CAD build for the part. Positions are in the model's coordinates, mm. Face numbers are marked on the shaded views. A direction names the side the tool comes from. Coordinates: 2 decimals unless noted, no trailing zeros. Order: outer loops, then holes, each group sorted by start corner. A loop starts at its lowest first (then second) coordinate and runs counter-clockwise, first axis right, second up. Notation, with made-up numbers: M 56,-24 L 71,-24 A32 cw 71,2 Z; hole C 89.25,-21 d5. An arc over 180 degrees is marked long. One line per item, written item: value.
Autodesk Inventor part; units mm, degrees
ref_plane "YZ Plane" through (0, 0, 0) normal (1, 0, 0) x (0, 1, 0)
ref_plane "XZ Plane" through (0, 0, 0) normal (0, 1, 0) x (-1, 0, 0)
ref_plane "XY Plane" through (0, 0, 0) normal (0, 0, 1) x (1, 0, 0)
sketch "Sketch1" plane through (0, 0, 0) normal (0, 0, 1) x (1, 0, 0)
  line L0 (0, 0) -> (82.55, 0)
  line L1 (82.55, 0) -> (82.55, 123.825)
  line L2 (82.55, 123.825) -> (0, 123.825)
  line L3 (0, 123.825) -> (0, 0)
  arc A0 (73.025, 123.825) -> (0, 6.35) centre (216.4664, -46.7758) ccw
  point P0 (60.325, 123.825)
  dimension "d0" = 82.55
  dimension "d1" = 123.825
  dimension "d5" = 9.525
  dimension "d6" = 6.35
extrude "Extrusion1" add sketch "Sketch1" along normal mid plane 46.0375 contours L3 A0 L2 L1 L0
sketch "Sketch3" plane through (0, 0, 23.0187) normal (-1, 0, 0) x (0, 0, 1)
  line L0 (-39.6875, 117.475) -> (-6.35, 117.475)
  line L1 (-6.35, 117.475) -> (-6.35, 3.175)
  line L2 (-6.35, 3.175) -> (-39.6875, 3.175)
  line L3 (-39.6875, 3.175) -> (-39.6875, 117.475)
  line L4 (0, 6.35) -> (0, 123.825)
  line L5 (-46.0375, 123.825) -> (0, 123.825)
  point P0 (-23.0187, 0)
  dimension "d9" = 33.3375
  dimension "d10" = 114.3
  dimension "d11" = 6.35
  dimension "d12" = 6.35
extrude "Extrusion2" cut sketch "Sketch3" along normal mid plane 158.75
sketch "Sketch4" plane through (79.375, 0, 23.0187) normal (-1, 0, 0) x (0, 0, 1)
  line L0 (-39.6875, 117.475) -> (-6.35, 117.475)
  line L1 (-39.6875, 117.475) -> (-6.35, 117.475)
  line L2 (-23.0188, 117.475) -> (-23.0188, 92.075)
  line L3 (-29.3688, 98.425) -> (-16.6688, 98.425)
  line L4 (-16.6688, 98.425) -> (-16.6688, 85.725)
  line L5 (-16.6688, 85.725) -> (-29.3688, 85.725)
  line L6 (-29.3688, 85.725) -> (-29.3688, 98.425)
  line L7 (-29.3688, 98.425) -> (-16.6688, 85.725) construction
  line L8 (-16.6688, 98.425) -> (-29.3688, 85.725) construction
  point P0 (-23.0187, 0)
  dimension "d26" = 25.4
  dimension "d27" = 12.7
  dimension "d28" = 12.7
extrude "Extrusion3" cut sketch "Sketch4" against normal through all
sketch "Sketch5" plane through (0, 3.175, 16.6688) normal (0, 1, 0) x (1, 0, 0)
  line L0 (60.325, 26.9875) -> (22.225, 26.9875)
  line L1 (22.225, 26.9875) -> (22.225, 3.175)
  line L2 (22.225, 3.175) -> (60.325, 3.175)
  line L3 (60.325, 3.175) -> (60.325, 26.9875)
  line L4 (65.7954, 33.3375) -> (0, 33.3375)
  line L5 (0, 0) -> (65.7954, 0)
  line L6 (0, 0) -> (0, 33.3375)
  point P0 (0, 16.6688)
  dimension "d20" = 6.35
  dimension "d21" = 3.175
  dimension "d22" = 22.225
  dimension "d23" = 38.1
extrude "Extrusion4" cut sketch "Sketch5" against normal blind 63.5
sketch "Sketch6" plane through (73.025, 123.825, 23.0187) normal (0, 1, 0) x (1, 0, 0)
  line L0 (9.525, 46.0375) -> (9.525, 0)
  line L1 (-73.025, 0) -> (9.525, 0)
  line L2 (9.525, 46.0375) -> (-7.684, 46.0375)
  line L3 (-7.684, 46.0375) -> (-7.684, 0)
  line L4 (-7.684, 0) -> (9.525, 0)
  line L5 (9.525, 0) -> (9.525, 46.0375)
  point P0 (-73.025, 23.0187)
extrude "Extrusion5" cut sketch "Sketch6" against normal blind 3.175
sketch "Sketch7" plane through (0, 0, 23.0187) normal (0, 0, 1) x (1, 0, 0)
  line L0 (82.55, 120.65) -> (82.55, 0)
  line L1 (0, 0) -> (82.55, 0)
  line L2 (82.55, 0) -> (82.55, 120.65)
  line L3 (82.55, 120.65) -> (0, 120.65)
  line L4 (0, 120.65) -> (0, 0)
extrude "Extrusion6" cut sketch "Sketch7" against normal blind 3.175
sketch "Sketch8" plane through (0, 0, -23.0187) normal (0, 0, -1) x (-1, 0, 0)
  line L0 (0, 0) -> (0, 6.35)
  line L1 (-82.55, 120.65) -> (-82.55, 0)
  line L2 (0, 0) -> (-82.55, 0)
  line L3 (-82.55, 0) -> (-82.55, 120.65)
  line L4 (-82.55, 120.65) -> (0, 120.65)
  line L5 (0, 120.65) -> (0, 0)
extrude "Extrusion7" cut sketch "Sketch8" against normal blind 3.175
properties part number "Pi Chassis"
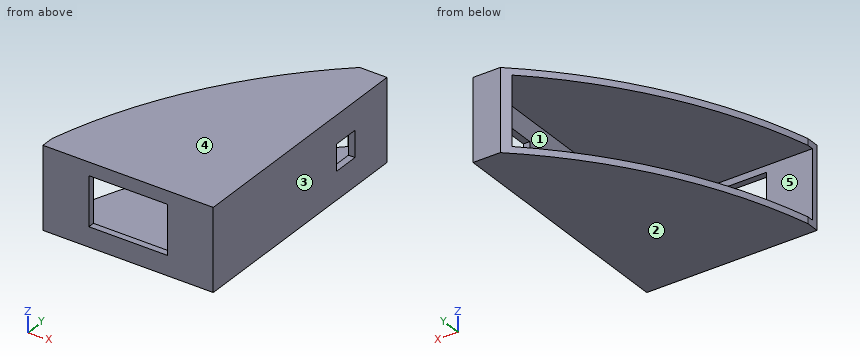
Q1. Slice it at A-A (z = -3). List the corners of the cut face in (x, y) (3 decimals).
Recorded:
outline: M 0,0 L 22.225,0 L 22.225,3.175 L 0,3.175 Z; M 60.325,0 L 82.55,0 L 82.55,85.725 L 79.375,85.725 L 79.375,3.175 L 60.325,3.175 Z; M 65.795,117.475 L 79.375,117.475 L 79.375,98.425 L 82.55,98.425 L 82.55,120.65 L 69.332,120.65 A222.89 ccw Z
Q2. Which spindle directions (+Z, -Z, +X, -X, +Y, -Y) get a long thin tool onto all of the face, cutting with end or side? Do the marked faces 1 and 2. Say none if no direction does.
Recorded:
face 1: -X
face 2: -Z, +X, -X, +Y, -Y
Q3. Slice it at B-B (x = 29.5). List the corners of the cut face in (y, z) (3 decimals).
Recorded:
outline: M 0,-19.844 L 74.565,-19.844 L 74.565,-16.669 L 3.175,-16.669 L 3.175,-10.319 L 0,-10.319 Z; M 0,13.494 L 3.175,13.494 L 3.175,16.669 L 74.565,16.669 L 74.565,19.844 L 0,19.844 Z
Q4. Slice it at C-C (y = 89.5). List the corners of the cut face in (x, z) (3 decimals).
Recorded:
outline: M 40.089,-19.844 L 82.55,-19.844 L 82.55,-6.35 L 79.375,-6.35 L 79.375,-16.669 L 40.089,-16.669 Z; M 40.089,16.669 L 79.375,16.669 L 79.375,6.35 L 82.55,6.35 L 82.55,19.844 L 40.089,19.844 Z
Q5. Slice it at D-D (x = 63.5). List the corners of the cut face in (y, z) (3 decimals), plus the area to 3 significant figures.
Recorded:
outline: M 0,-19.844 L 115.339,-19.844 L 115.339,-16.669 L 3.175,-16.669 L 3.175,16.669 L 115.339,16.669 L 115.339,19.844 L 0,19.844 Z
area: 838 mm^2
Q6. Drill centre lines: line 1 along Z through (x, y) = (15, 11); line 2 along Y through (x, z) = (72, 15) (3 decimals); line 3 along X through (y, z) = (27.5, -3.5) (3 decimals). Where is each one in solid material? Low to high.
Recorded:
line 1: z = -19.84 to -16.67, 16.67 to 19.84
line 2: y = 0 to 3.175, 117.475 to 120.65
line 3: x = 79.375 to 82.55
Q7. Pin check, flat tips, straight feed: pin 1 Ø1 at (x, z) = (57, -9.5) entering from -Y; pin 2 Ø3 at (x, z) = (20.5, -10.5) entering from +Y (3 decimals); pin 3 Ø10 at (y, z) = (86.5, 2) entering from -X (3 decimals). Stop position of each tip, or through.
Recorded:
pin 1: passes through
pin 2: stops at y = 3.175
pin 3: stops at x = 79.375
Q8. Mould opens along Z. For the marked faces 3, 4 and 5 say: released by +Z, released by -Z, zero draft, split by the parting line, or undercut.
Recorded:
face 3: zero draft
face 4: released by +Z
face 5: undercut
